Input: dimensioned drawing with shaded views. Units: mm. Origin: part minimum x, y, z. A direction names the side the tool comes from. Round coordinates to 2 decimals unless told otherwise and drop trailing zeros. Loops run counter-clockwise (first coordinate to the right, second up) from the corner with the lowest first, then second, coordinate; pieces in that order, holes last. Notation, with made-up numbers: (-23.75, 6) - (34.25, 6) arc R23 ccw to (34.25, 22) - close; hole circle Ø7 at (-28.75, -1.5). An arc over 180 degrees is marked (long way). Answer as a JSON object with one key per item and string values. Group by question number.
Item 1: Draft query along X for the marked faces 1, 2 and 3. Return one class per face: released by +X, released by -X, zero draft, split by the parting line, or undercut.
Item 2: First-contact query: pin 1 (6.5 mm diameter, centred on y = 31, z = 5.5, fed in from +X). Flat tip, straight axial feed; report the tip coordinate or a pass-through.
Item 3: Section B-B (y = 10). Return the cut outline in (x, z), plus the area to 3 significant figures.
Item 4: Line query: line 1 (X direction, y = 22, z = 6.5); line 2 (Y direction, x = 9.5, z = 5); line 3 (X direction, y = 29, z = 21). Output: solid intervals per line, ascending.
Item 5: Section C-C (x = 4). Return the cut outline in (y, z), plus the area to 3 significant figures.
Item 6: Reachability of the marked faces 4 and 5 from +Z, -Z, +X, -X, +Y, -Y: full face, straight path, thin tool, end or side. Return the list, or none.
Item 7: Section A-A (z = 20.5). Return the cut outline in (x, y), plus the area to 3 significant figures.
Item 8: Section D-D (z = 5.5). Return the cut outline in (x, y).
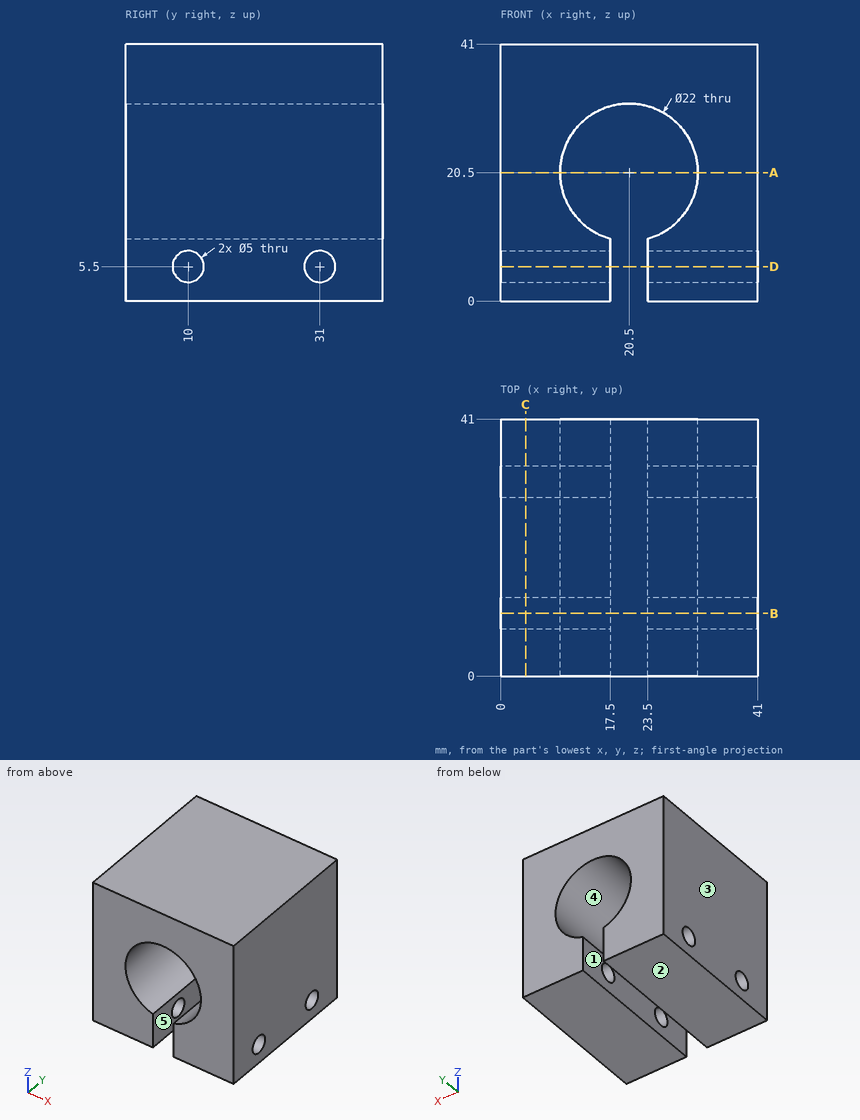
Values:
{
 "1": {"face 1": "undercut", "face 2": "zero draft", "face 3": "released by -X"},
 "2": {"pin 1": "stops at x = 41"},
 "3": {"outline": "(0, 0) - (17.5, 0) - (17.5, 3) - (0, 3) - close; (0, 8) - (17.5, 8) - (17.5, 9.92) arc R11 cw (long way) to (23.5, 9.92) - (23.5, 8) - (41, 8) - (41, 41) - (0, 41) - close; (23.5, 0) - (41, 0) - (41, 3) - (23.5, 3) - close", "area": "1,070 mm^2"},
 "4": {"line 1": "x = 0 to 17.5, 23.5 to 41", "line 2": "y = 0 to 7.55, 12.45 to 28.55, 33.45 to 41", "line 3": "x = 0 to 9.51, 31.49 to 41"},
 "5": {"outline": "(0, 0) - (41, 0) - (41, 41) - (0, 41) - close; hole circle Ø5 at (10, 5.5); hole circle Ø5 at (31, 5.5)", "area": "1,640 mm^2"},
 "6": {"face 4": "+Y, -Y", "face 5": "-Z, +Y, -Y"},
 "7": {"outline": "(0, 0) - (9.5, 0) - (9.5, 41) - (0, 41) - close; (31.5, 0) - (41, 0) - (41, 41) - (31.5, 41) - close", "area": "779 mm^2"},
 "8": {"outline": "(0, 0) - (17.5, 0) - (17.5, 7.5) - (0, 7.5) - close; (0, 12.5) - (17.5, 12.5) - (17.5, 28.5) - (0, 28.5) - close; (0, 33.5) - (17.5, 33.5) - (17.5, 41) - (0, 41) - close; (23.5, 0) - (41, 0) - (41, 7.5) - (23.5, 7.5) - close; (23.5, 12.5) - (41, 12.5) - (41, 28.5) - (23.5, 28.5) - close; (23.5, 33.5) - (41, 33.5) - (41, 41) - (23.5, 41) - close"}
}
